Autodesk Inventor part; units mm, degrees
ref_plane "작업 평면1" through (17, 2, -0.9) normal (1, 0, 0) x (0, 0, -1)
ref_plane "YZ Plane" through (0, 0, 0) normal (1, 0, 0) x (0, 1, 0)
ref_plane "XZ Plane" through (0, 0, 0) normal (0, 1, 0) x (-1, 0, 0)
sketch "스케치1" plane through (0, 0, 0) normal (0, 0, 1) x (1, 0, 0)
  line L0 (0, 0) -> (17, 0)
  line L1 (17, 0) -> (17, 8)
  line L2 (17, 8) -> (0, 8)
  line L3 (0, 8) -> (0, 0)
  line L4 (0, 4.8) -> (17, 4.8)
  line L5 (15, 8) -> (15, 0)
  dimension "d0" = 17
  dimension "d1" = 8
  dimension "d3" = 4.8
  dimension "d4" = 15
extrude "돌출1" add sketch "스케치1" along normal mid plane 1.8
sketch "스케치3" plane through (0, 0, 0.9) normal (-1, 0, 0) x (0, 0, 1)
  line L0 (-1.8, 0) -> (0, 0)
  line L1 (-1.8, 0) -> (-1.8, 8)
  line L2 (-1.7, 7.7) -> (-0.1, 7.7)
  line L3 (-0.1, 7.7) -> (-0.1, 0.3)
  line L4 (-0.1, 0.3) -> (-1.7, 0.3)
  line L5 (-1.7, 0.3) -> (-1.7, 7.7)
  line L6 (-1.8, 8) -> (0, 8)
  line L7 (0, 8) -> (0, 0)
  point P0 (-0.9, 0)
  dimension "d11" = 0.3
  dimension "d12" = 0.3
  dimension "d13" = 0.1
  dimension "d14" = 0.1
sketch "스케치5" plane through (0, 0, -0.9) normal (0, 0, -1) x (-1, 0, 0)
  line L0 (0, 0) -> (0, 8)
  line L1 (-17, 0) -> (0, 0)
  line L2 (-9.9, 6.5) -> (-7.1, 6.5)
  line L3 (-7.1, 6.5) -> (-7.1, 4)
  line L4 (-7.1, 4) -> (-9.9, 4)
  line L5 (-9.9, 4) -> (-9.9, 6.5)
  line L6 (-17, 8) -> (-17, 0)
  line L7 (0, 8) -> (-17, 8)
  dimension "d21" = 2.8
  dimension "d22" = 2.5
  dimension "d24" = 1.5
  dimension "d25" = 7.1
extrude "돌출3" add sketch "스케치5" along normal blind 1 contours L2 L3 L4 L5
sketch "스케치6" plane through (0, 0, -1.9) normal (0, 0, -1) x (-1, 0, 0)
  line L0 (-9, 5.75) -> (-8, 5.75)
  line L1 (-8, 5.75) -> (-8, 4.75)
  line L2 (-8, 4.75) -> (-9, 4.75)
  line L3 (-9, 4.75) -> (-9, 5.75)
  line L4 (-9, 5.75) -> (-8, 4.75) construction
  line L5 (-8, 5.75) -> (-9, 4.75) construction
  line L6 (0, 8) -> (-17, 8)
  line L7 (0, 0) -> (0, 8)
  point P0 (-8.5, 5.25)
  dimension "d28" = 1
  dimension "d29" = 1
  dimension "d30" = 2.75
  dimension "d31" = 8.5
sketch "스케치7" plane through (7.1, 6.5, -0.9) normal (0, 1, 0) x (1, 0, 0)
  line L0 (0, 0) -> (0, 1)
  line L1 (0.1, 0.2799) -> (2.7, 0.2799)
  line L2 (2.7, 0.2799) -> (2.7, 0.7799)
  line L3 (2.7, 0.7799) -> (0.1, 0.7799)
  line L4 (0.1, 0.7799) -> (0.1, 0.2799)
  point P0 (-7.1, -0.9)
  point P1 (2.8, 0)
  dimension "d32" = 0.5
  dimension "d33" = 2.6
  dimension "d34" = 0.1
extrude "돌출4" cut sketch "스케치7" against normal blind 2.49
extrude "돌출5" cut sketch "스케치6" against normal blind 0.5
sketch "스케치8" plane through (0, 8, 0.9) normal (0, 1, 0) x (1, 0, 0)
  line L0 (17, 1.8) -> (0, 1.8)
  line L1 (17, 0) -> (0, 0)
  line L2 (11, 1.8) -> (6, 1.8)
  line L3 (6, 1.8) -> (6, 0)
  line L4 (6, 0) -> (11, 0)
  line L5 (11, 0) -> (11, 1.8)
  line L6 (17, 0) -> (17, 1.8)
  point P0 (0, 0.9)
  point P1 (11, 0)
  dimension "d39" = 5
  dimension "d40" = 6
extrude "돌출6" add sketch "스케치8" along normal blind 0.5 contours L5 L1 L3 L0
sketch "스케치9" plane through (0, 0, -0.9) normal (0, 0, -1) x (-1, 0, 0)
  line L0 (-10, 8.3) -> (-7, 8.3)
  line L1 (-7, 8.3) -> (-7, 8.1)
  line L2 (-7, 8.1) -> (-10, 8.1)
  line L3 (-10, 8.1) -> (-10, 8.3)
  line L4 (-11, 8) -> (-11, 8.5)
  line L5 (-11, 8.5) -> (-6, 8.5)
  point P0 (0, 0)
  dimension "d43" = 0.2
  dimension "d44" = 3
  dimension "d45" = 1
  dimension "d46" = 0.2
extrude "돌출7" cut sketch "스케치9" against normal blind 6
fillet "모깎기1" radius 2 4 edges at (11, 8.5, 0) (6, 8.5, 0) (11, 8, 0) (6, 8, 0)
fillet "모깎기3" radius 0.5 2 edges at (0, 0, 0) (0, 8, 0)
ref_plane "작업 평면1" through (17, 2, -0.9) normal (1, 0, 0) x (0, 0, -1)
sketch "스케치10" plane through (17, 2, -0.9) normal (1, 0, 0) x (0, 0, -1)
  line L0 (-1.7, 5.7) -> (-0.1, 5.7)
  line L1 (-0.1, 5.7) -> (-0.1, -1.7)
  line L2 (-0.1, -1.7) -> (-1.7, -1.7)
  line L3 (-1.7, -1.7) -> (-1.7, 5.7)
  line L4 (-1.8, 4) -> (-1.8, 6)
  line L5 (0, 4) -> (0, 0)
  line L6 (0, 6) -> (-1.8, 6)
  line L7 (-1.8, -2) -> (0, -2)
  point P0 (-0.9, -2)
  dimension "d52" = 0.1
  dimension "d53" = 0.1
  dimension "d54" = 0.3
  dimension "d55" = 0.3
extrude "돌출8" cut sketch "스케치10" against normal blind 16.5
properties part number "bobecase"
Geometry: final body of the model. Coordinates: model frame, mm. A direction names the side the tool comes from. Coordinates: 2 decimals unless noted, no trailing zeros. Order: outer loops, then holes, each group sorted by start corner. A loop starts at its lowest first (then second) coordinate and runs counter-clockwise, first axis right, second up.
(1) Material intervals for probe 1 along Y at (x, z) = (2.75, 0.55); probe 2 along Y at (x, z) = (5.75, 0.2); probe 3 along X at (y, z) = (1.5, -0.5), sorted ascending.
(2) Section query A-A (x = 13.5). Return the cut outline in (y, z).
(3) Draft query along X for faces 1 (the face through (8, 8.1, 0)), 2 (the face through (0.5, 4, 0)), 3 (the face through (0, 4, 0)). Return one class per face: pulls with the +X half, pulls with the -X half, needs draft (parallel to the pull), parting line crosses it, or undercut.
(4) Section query B-B (y = 5.5). Return the cut outline in (x, z).
(5) Access query for faces 4 (the face through (9, 8.3, 0)), 5 (the face through (3, 8, 0)), 6 (the face through (9, 5, -0.8)). Directions: +Z, -Z, +X, -X, +Y, -Y. A direction counts if a zero-diameter tool reaches every point of the face in a straight line with its end or side. Return the directions, or none.
(6) First-contact query: pin 1 (1.4 mm diameter, centred on x = 2.5, z = 0, fed in from +Y); pin 2 (1.1 mm diameter, centred on y = 5.5, z = -1.5, fed in from -X); pin 3 (1 mm diameter, centred on x = 9, z = -1.5, fed in from +Y). Flat tips, straight axial feed; report the tip coordinate or a pass-through.
(7) Section query D-D (y = 3.25). Return the cut outline in (x, z).
(8) Section query C-C (z = -0.2). Return the cut outline in (x, y).
Solution:
1. probe 1: y = 0 to 0.3, 7.7 to 8
1. probe 2: y = 0 to 0.3, 7.7 to 8.3
1. probe 3: x = 0 to 0.5
2. outline: (0, -0.9) - (8, -0.9) - (8, 0.9) - (0, 0.9) - close; hole (0.3, -0.8) - (7.7, -0.8) - (7.7, 0.8) - (0.3, 0.8) - close
3. face 1: undercut
3. face 2: pulls with the +X half
3. face 3: pulls with the -X half
4. outline: (0, -0.9) - (7.1, -0.9) - (7.1, -1.9) - (8, -1.9) - (8, -1.68) - (7.2, -1.68) - (7.2, -1.18) - (9.8, -1.18) - (9.8, -1.68) - (9, -1.68) - (9, -1.9) - (9.9, -1.9) - (9.9, -0.9) - (17, -0.9) - (17, -0.8) - (0.5, -0.8) - (0.5, 0.8) - (17, 0.8) - (17, 0.9) - (0, 0.9) - close
5. face 4: +Z, -Z
5. face 5: +Z, -Z, -X, +Y
5. face 6: +X
6. pin 1: stops at y = 8
6. pin 2: stops at x = 7.1
6. pin 3: stops at y = 6.5
7. outline: (0, -0.9) - (17, -0.9) - (17, -0.8) - (0.5, -0.8) - (0.5, 0.8) - (17, 0.8) - (17, 0.9) - (0, 0.9) - close
8. outline: (0, 0.5) arc R0.5 ccw to (0.5, 0) - (17, 0) - (17, 0.3) - (0.5, 0.3) - (0.5, 7.7) - (17, 7.7) - (17, 8) - (12.32, 8) arc R2 cw to (11.35, 8.25) arc R2 ccw to (10.39, 8.5) - (6.61, 8.5) arc R2 ccw to (5.65, 8.25) arc R2 cw to (4.68, 8) - (0.5, 8) arc R0.5 ccw to (0, 7.5) - close; hole (7, 8.1) - (10, 8.1) - (10, 8.3) - (7, 8.3) - close
